Can you work these out from the drawing? Everything is in mm from the part's minimum corner. Round coordinates to 2 decimals unless told otherwise and drop trailing zeros. Loops run counter-clockwise (first coordinate to the right, second up) from the corner with the lowest first, then second, coordinate; pieces in that order, holes last. Notation, with made-up numbers: (19, 10) -> (62, 10) arc R8 cw to (62, 16) -> close; hole circle Ø6 at (3.5, 3). An arc over 180 degrees is marked (long way). One line per item, written item: value.
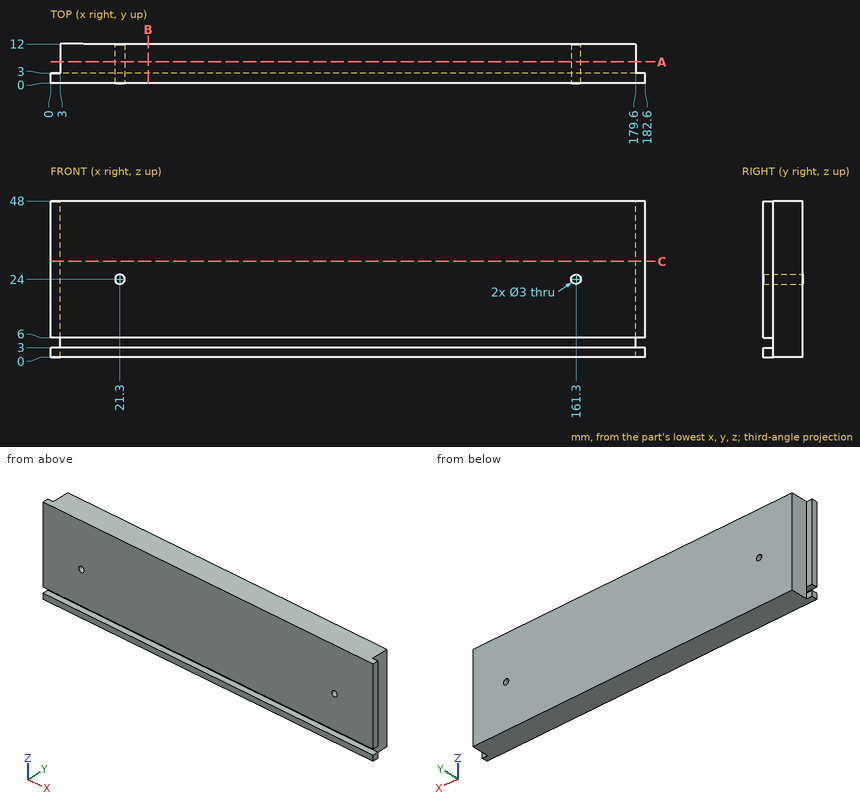
(1) Imagine slicing it at A-A on y = 6.5. Write out the boundary of the cut face in (x, z), then the cut area to 3 significant figures.
Results below:
outline: (3, 0) -> (179.6, 0) -> (179.6, 48) -> (3, 48) -> close; hole circle Ø3 at (21.3, 24); hole circle Ø3 at (161.3, 24)
area: 8,460 mm²
(2) Please list where these lines run through material, in increasing order: L1, parallel to Z at x = 161.3, y = 7; L2, parallel to X at y = 4, z = 24.5; L3, parallel to Z at x = 155, y = 1.75.
Results below:
L1: z = 0 to 22.5, 25.5 to 48
L2: x = 3 to 19.89, 22.71 to 159.89, 162.71 to 179.6
L3: z = 0 to 3, 6 to 48
(3) For pin 1 Ø3 at (y, z) = (8, 8.5) entering from -X; pin 2 Ø1.5 at (x, z) = (1, 26) entering from +Y; pin 3 Ø1 at (y, z) = (9, 43) entering from +X, each with a flat end and sliding along its axis, tell me the tip position at first contact or that it passes through.
Results below:
pin 1: stops at x = 3
pin 2: stops at y = 3
pin 3: stops at x = 179.6
(4) Imagine slicing it at C-C on z = 29.5. Write out the boundary of the cut face in (x, y).
Results below:
outline: (0, 0) -> (182.6, 0) -> (182.6, 3) -> (179.6, 3) -> (179.6, 12) -> (3, 12) -> (3, 3) -> (0, 3) -> close
(5) Imagine slicing it at B-B on x = 30. Write out the boundary of the cut face in (y, z), then the cut area to 3 significant figures.
Results below:
outline: (0, 0) -> (12, 0) -> (12, 48) -> (0, 48) -> (0, 6) -> (3, 6) -> (3, 3) -> (0, 3) -> close
area: 567 mm²
